Autodesk Inventor part; units mm, degrees
ref_plane "YZ Plane" through (0, 0, 0) normal (1, 0, 0) x (0, 1, 0)
ref_plane "XZ Plane" through (0, 0, 0) normal (0, 1, 0) x (-1, 0, 0)
ref_plane "XY Plane" through (0, 0, 0) normal (0, 0, 1) x (1, 0, 0)
sketch "Sketch1" plane through (0, 0, 0) normal (0, 1, 0) x (-1, 0, 0)
  line L0 (0, 0) -> (55, 0)
  line L1 (55, 0) -> (55, -55)
  line L2 (55, -55) -> (0, -55)
  line L3 (0, -55) -> (0, 0)
  line L4 (47.55, -7.45) -> (7.45, -7.45) construction
  line L5 (7.45, -7.45) -> (7.45, -47.55) construction
  line L6 (7.45, -47.55) -> (47.55, -47.55) construction
  line L7 (47.55, -47.55) -> (47.55, -7.45) construction
  circle A0 centre (47.55, -47.55) radius 2.6
  circle A1 centre (7.45, -47.55) radius 2.6
  circle A2 centre (27.5, -7.45) radius 3.8
  line L8 (0, -17.5) -> (17.5, 0)
  line L9 (37.5, 0) -> (55, -17.5)
  dimension "d0" = 55
  dimension "d1" = 55
  dimension "d2" = 40.1
  dimension "d3" = 40.1
  dimension "d6" = 5.2
  dimension "d7" = 5.2
  dimension "d8" = 7.45
  dimension "d9" = 7.45
  dimension "d14" = 7.6
  dimension "d55" = 20
  dimension "d56" = 10
extrude "Extrusion1" add sketch "Sketch1" along normal blind 3 contours L0 L9 L1 L2 L3 L8
fillet "Fillet1" radius 5 6 edges at (-55, 1.5, -55) (0, 1.5, -55) (-55, 1.5, -17.5) (-37.5, 1.5, 0) (-17.5, 1.5, 0) (0, 1.5, -17.5)
sketch "Sketch2" plane through (0, 0, 0) normal (0, -1, 0) x (1, 0, 0)
  line L0 (-17.5, -40) -> (-37.5, -40)
  line L1 (-37.5, -40) -> (-37.5, -20)
  line L2 (-37.5, -20) -> (-17.5, -20)
  line L3 (-17.5, -20) -> (-17.5, -40)
  line L4 (-5, -55) -> (-50, -55)
  line L5 (-17.5, -40) -> (-37.5, -40)
  line L6 (-37.5, -47) -> (-37.5, -55)
  line L7 (-37.5, -55) -> (-17.5, -55)
  line L8 (-17.5, -55) -> (-17.5, -47)
  line L9 (0, -19.5711) -> (0, -50)
  line L10 (-55, -50) -> (-55, -19.5711)
  line L11 (-10.5, -40) -> (0, -40)
  line L12 (0, -40) -> (0, -20)
  line L13 (0, -20) -> (-17.5, -20)
  line L14 (-17.5, -20) -> (-17.5, -40)
  line L15 (-44.5, -40) -> (-55, -40)
  line L16 (-55, -40) -> (-55, -20)
  line L17 (-55, -20) -> (-37.5, -20)
  line L18 (-37.5, -20) -> (-37.5, -40)
  arc A0 (-10.5, -40) -> (-17.5, -47) centre (-10.5, -47) ccw
  arc A1 (-37.5, -47) -> (-44.5, -40) centre (-44.5, -47) ccw
  point P0 (0, -40)
  point P1 (-17.5, -55)
  dimension "d68" = 20
  dimension "d69" = 20
  dimension "d70" = 55
  dimension "d71" = 17.5
  dimension "d72" = 15
  dimension "d73" = 7
extrude "Extrusion8" add sketch "Sketch2" along normal blind 20 contours L3 L13 L9 L11 A0 L8 L4 L6 A1 L15 L10 L17 L1 L0
sketch "Sketch6" plane through (-55, 0, -50) normal (-1, 0, 0) x (0, 0, 1)
  line L0 (10, -20) -> (30, -20) construction
  line L1 (10, 0) -> (30, 0) construction
  line L2 (10, -20) -> (30, 0) construction
  circle A0 centre (20, -10) radius 3
  point P0 (50, 0)
  dimension "d44" = 6
extrude "Extrusion9" cut sketch "Sketch6" against normal through all
sketch "Sketch7" plane through (-55, 0, -50) normal (-1, 0, 0) x (0, 0, 1)
  circle A0 centre (20, -10) radius 3
  circle A1 centre (20, -10) radius 5.5
  point P0 (50, 0)
  dimension "d47" = 11
extrude "Extrusion10" cut sketch "Sketch7" against normal blind 11 contours A0 | A1
sketch "Sketch8" plane through (0, 0, -50) normal (1, 0, 0) x (0, 0, -1)
  line L0 (-30, 0) -> (-30, -20) construction
  line L1 (-10, 0) -> (-30, 0) construction
  line L2 (-30, -20) -> (-10, 0) construction
  circle A0 centre (-20, -10) radius 5.5
  circle A1 centre (-20, -10) radius 5.5 construction
  point P0 (-50, 0)
extrude "Extrusion11" cut sketch "Sketch8" against normal blind 11
chamfer "Chamfer3" distance 10 angle 45 2 edges at (-55, -20, -30) (0, -20, -30)
sketch "Sketch11" plane through (-5, 3, -55) normal (0, 0, -1) x (-1, 0, 0)
  line L0 (32.5, -23) -> (12.5, -23) construction
  line L1 (12.5, -23) -> (32.1967, -3) construction
  line L2 (33.9645, -3) -> (30.4289, -3) construction
  circle A0 centre (22.3483, -13) radius 2.5
  point P0 (-5, -3)
  dimension "d74" = 5
extrude "Extrusion14" cut sketch "Sketch11" against normal blind 12.5
chamfer "Chamfer4" distance 3 angle 45 1 edges at (-27.5, -20, -55)
fillet "Fillet2" radius 2 6 edges at (-55, -5, -40) (-55, -5, -20) (0, -5, -20) (0, -5, -40) (-37.5, -8.5, -55) (-17.5, -8.5, -55)
equation "\"d1\" = d0"
equation "\"d3\" = d2"
equation "\"d8\" = -0.5 * d2 + 0.5 * d0"
equation "\"d9\" = -0.5 * d3 + 0.5 * d1"
equation "\"d71\" = -0.5 * d68 + 0.5 * d70"
properties part number "Gantry Plate" material "PC/ABS Plastic"
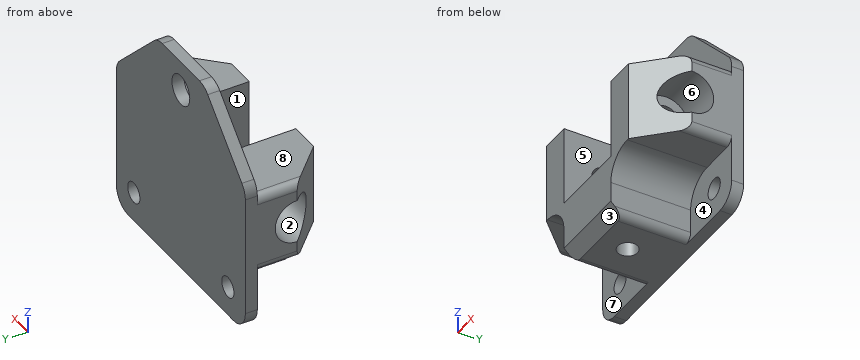
Geometry check sheet. Reference: the model listing, model coordinates, mm. Face numbers are marked on the shaded views. A direction names the side the tool comes from. Coordinates: 2 decimals unless noted, no trailing zeros. Order: outer loops, then holes, each group sorted by start corner. A loop starts at its lowest first (then second) coordinate and runs counter-clockwise, first axis right, second up. Notation, with made-up numbers: M -36.5,31.5 L -19.5,31.5 A23 ccw -19.5,58.5 Z; hole C 75,-25 d9. An arc over 180 degrees is marked long. Answer as a JSON object with one key per item and string values.
Q1. Cross-section at A-A on x = -8. Record the cut outline in (y, z).
Results are:
{"outline": "M -18,-40 L 0,-40 L 0,-45.01 L 3,-45.01 L 3,-9.5 L 0,-9.5 L 0,-20 L -18,-20 Z; M 0,-55 L 3,-55 L 3,-50.09 L 0,-50.09 Z; hole C -10,-30 d11"}
Q2. Release check for a two-part mould opening along Y. For the marked faces 1, 2 and 3 record: released by +Y, released by -Y, zero draft, split by the parting line, or undercut.
Results are:
{"face 1": "zero draft", "face 2": "undercut", "face 3": "released by -Y"}
Q3. Depth check by flat-ended pin: pin 1 Ø1.8 at (y, z) = (-8.5, -49.5) entering from +X; pin 2 Ø6 at (x, y) = (-29.5, -7) entering from +Z; pin 3 Ø1 at (x, z) = (-41.5, -41.5) entering from -Y; pin 4 Ø3.5 at (y, z) = (-10, -30) entering from -X. Enter the tip coordinate at first touch or a pass-through.
Results are:
{"pin 1": "stops at x = -17.5", "pin 2": "stops at z = -40", "pin 3": "stops at y = 0", "pin 4": "passes through"}
Q4. Tool access check on the marked faces 4, 5, 6, 7 and 8. Record the directions out of +Z, -Z, +X, -X, +Y, -Y that give a thin tool (end or side, any length) a straight path to the whole face; none if there is none.
Results are:
{"face 4": "-Z, +X, -Y", "face 5": "+Z, -Y", "face 6": "+X", "face 7": "-Z, -X, -Y", "face 8": "+Z, +X, -X, -Y"}
Q5. Cross-section at D-D on y = -3.5. Record the cut outline in (x, z).
Results are:
{"outline": "M -55,-38 A2 ccw -53,-40 L -44.5,-40 A7 cw -37.5,-47 L -37.5,-53 A2 ccw -35.5,-55 L -19.5,-55 A2 ccw -17.5,-53 L -17.5,-47 A7 cw -10.5,-40 L -2,-40 A2 ccw 0,-38 L 0,-22 A2 ccw -2,-20 L -17.5,-20 L -17.5,-40 L -37.5,-40 L -37.5,-20 L -53,-20 A2 ccw -55,-22 Z"}
Q6. Cross-section at B-B on z = -30. Record the cut outline in (x, y).
Results are:
{"outline": "M -55,-4.5 L -44,-4.5 L -44,-7 L -37.5,-7 L -37.5,0 L -17.5,0 L -17.5,-7 L -11,-7 L -11,-4.5 L 0,-4.5 L 0,3 L -55,3 Z; M -49.5,-15.5 L -45,-20 L -37.5,-20 L -37.5,-13 L -44,-13 L -44,-15.5 Z; M -17.5,-20 L -10,-20 L -5.5,-15.5 L -11,-15.5 L -11,-13 L -17.5,-13 Z"}
Q7. Scan lines: line 1 (X direction, y = -0.25, z = -35.5); line 2 (Z direction, x = -7.45, y = 1.55); line 3 (Y direction, x = -14.5, z = -30). Record each from-to range of solid material in increasing order.
Results are:
{"line 1": "x = -55 to -37.5, -17.5 to 0", "line 2": "z = -55 to -50.15, -44.95 to -10.05", "line 3": "y = -20 to -13, -7 to 3"}
Q8. Cross-section at C-C on z = -7.45. Record the cut outline in (x, y), and give its area (3 significant figures).
Results are:
{"outline": "M -44.95,0 L -31.3,0 L -31.3,3 L -44.95,3 Z; M -23.7,0 L -10.05,0 L -10.05,3 L -23.7,3 Z", "area": "81.9 mm²"}
